Here's the drawing with two shaded views (mm, measured from the low corner). I have some questions. Give positions to 0.01 mm unless a question says otherwise; leave off trailing zeros. Use one line per item in the form item = value. Start each with the question number.
1) For pin 1 (2 mm diameter, centred on x = 71, y = 2, fed in from -Z), with a flat end and sliding along its axis, tell me the tip position at first contact or that it passes through.
2) Please list where these lines run through material, in increasing order: probe 1 along X at (y, z) = (8.5, 105.5); probe 2 along X at (y, z) = (7.25, 62).
3) Suppose I cut it at B-B, the plane x = 45. State how many separate pieces and enclosed holes the cut face has, and give its area (3 significant figures).
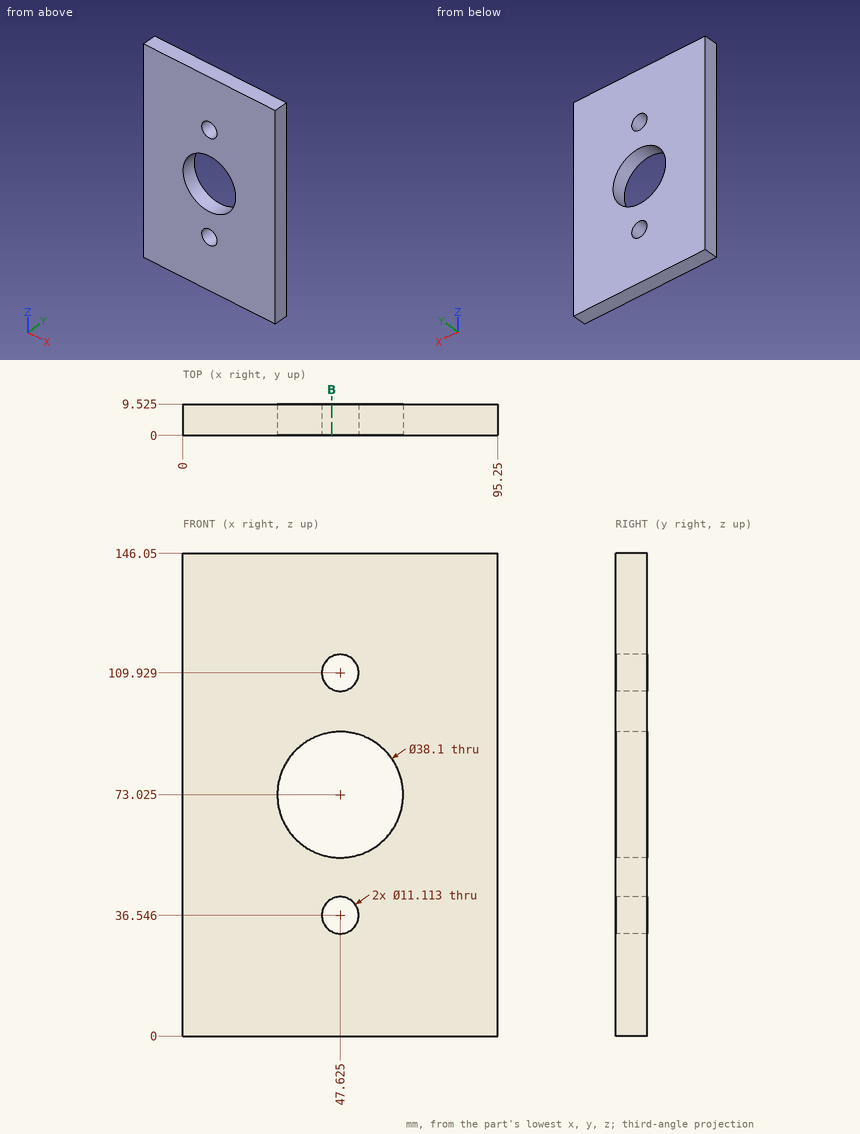
Result sheet:
q1.pin_1 = 0
q2.probe_1 = 0 to 44.27, 50.98 to 95.25
q2.probe_2 = 0 to 32.09, 63.16 to 95.25
q3.separate_pieces = 4
q3.enclosed_holes = 0
q3.area = 845 mm²
